Geometry check sheet. Reference: the model listing, model coordinates, mm. Face numbers are marked on the shaded views. A direction names the side the tool comes from. Coordinates: 2 decimals unless noted, no trailing zeros. Loops run counter-clockwise (first coordinate to the right, second up) from the corner with the lowest first, then second, coordinate; pieces in that order, holes last.
from build123d import *

# Parameters (mm, degrees)
F0_W     = 100
F0_H     = 80
F1_DEPTH = 25
F2_R     = 15
F3_DEPTH = 30
F4_R     = 15
F5_DEPTH = 25


with BuildPart() as f1:
    # F0 (on Top) → F1 (new body)
    with BuildSketch(Plane.XY):
        Rectangle(F0_W, F0_H)
    extrude(amount=F1_DEPTH)

    # F2 (on face) → F3 (join)
    with BuildSketch(Plane.XY.offset(25)):
        with Locations((-25, 0)):
            Circle(F2_R)
    extrude(amount=F3_DEPTH)

    # F4 (on face) → F5 (cut)
    with BuildSketch(Plane.XY.offset(25)):
        with Locations((25, 0)):
            Circle(F4_R)
    extrude(amount=-F5_DEPTH, mode=Mode.SUBTRACT)


solid = f1.part
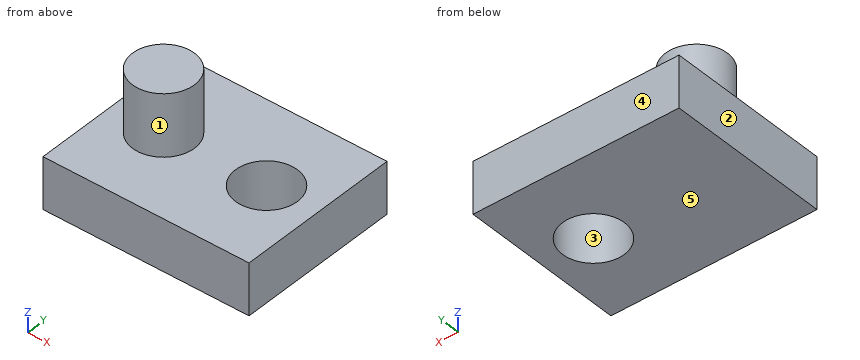
(1) Sectioned sample at C-C on x = -25. Record the cut outline in (y, z), and give its area (3 significant figures).
Findings:
outline: (-40, 0) - (40, 0) - (40, 25) - (15, 25) - (15, 55) - (-15, 55) - (-15, 25) - (-40, 25) - close
area: 2,900 mm2
(2) Sectioned sample at A-A on x = 25. Record the cut outline in (y, z), and give its area (3 significant figures).
Findings:
outline: (-40, 0) - (-15, 0) - (-15, 25) - (-40, 25) - close; (15, 0) - (40, 0) - (40, 25) - (15, 25) - close
area: 1,250 mm2
(3) Sectioned sample at D-D on z = 29.5. Record the cut outline in (x, y).
Findings:
outline: circle Ø30 at (-25, 0)
(4) Access from +Z, -Z, +X, -X, +Y, -Y to the whole of each face (thin tool, end or side, straight path). Record for the marked faces 1 and 2.
Findings:
face 1: +Z
face 2: +Z, -Z, -X, +Y, -Y
(5) Gauge pin test, flat ends, axial feed: pin 1 Ø1 at (y, z) = (-11.5, 46) entering from -X; pin 2 Ø3 at (x, y) = (38, 25.5) entering from +Z. Record the tip position at first contact, or that the pin passes through.
Findings:
pin 1: stops at x = -35.2
pin 2: stops at z = 25
(6) Scan lines: L1, parallel to Y at x = 25, z = 19.5; L2, parallel to Z at x = -2.5, y = -9.5; L3, parallel to Y at x = 15.5, z = 11.5. Record each from-to range of solid material in increasing order.
Findings:
L1: y = -40 to -15, 15 to 40
L2: z = 0 to 25
L3: y = -40 to -11.61, 11.61 to 40
(7) Sectioned sample at B-B on y = 12.5. Record the cut outline in (x, z).
Findings:
outline: (-50, 0) - (16.71, 0) - (16.71, 25) - (-16.71, 25) - (-16.71, 55) - (-33.29, 55) - (-33.29, 25) - (-50, 25) - close; (33.29, 0) - (50, 0) - (50, 25) - (33.29, 25) - close
(8) Draft check along Y on the marked faces 3, 4 and 5. Enter one of: +Y half, -Y half, draft (parallel to the pull), parting line (faces both ways), or undercut.
Findings:
face 3: undercut
face 4: +Y half
face 5: draft
